The figure shows three views and two pictorial views of one solid part (mm, origin at its lowest corner). Answer the questions. A direction names the side the tool comes from. Coordinates: 2 decimals unless noted, no trailing zeros. Write each loop counter-clockwise with the first axis right and the second up, starting at its lowest first coordinate (ties: lowest second). Pieces come first, ordered by that corner, then holes. Notation, with made-up numbers: M 36.25,59 L 51.25,59 A20 ccw 51.25,75 Z; hole C -18.5,71.25 d2. An arc over 180 degrees is marked long. Answer as CSV lines item,"result".
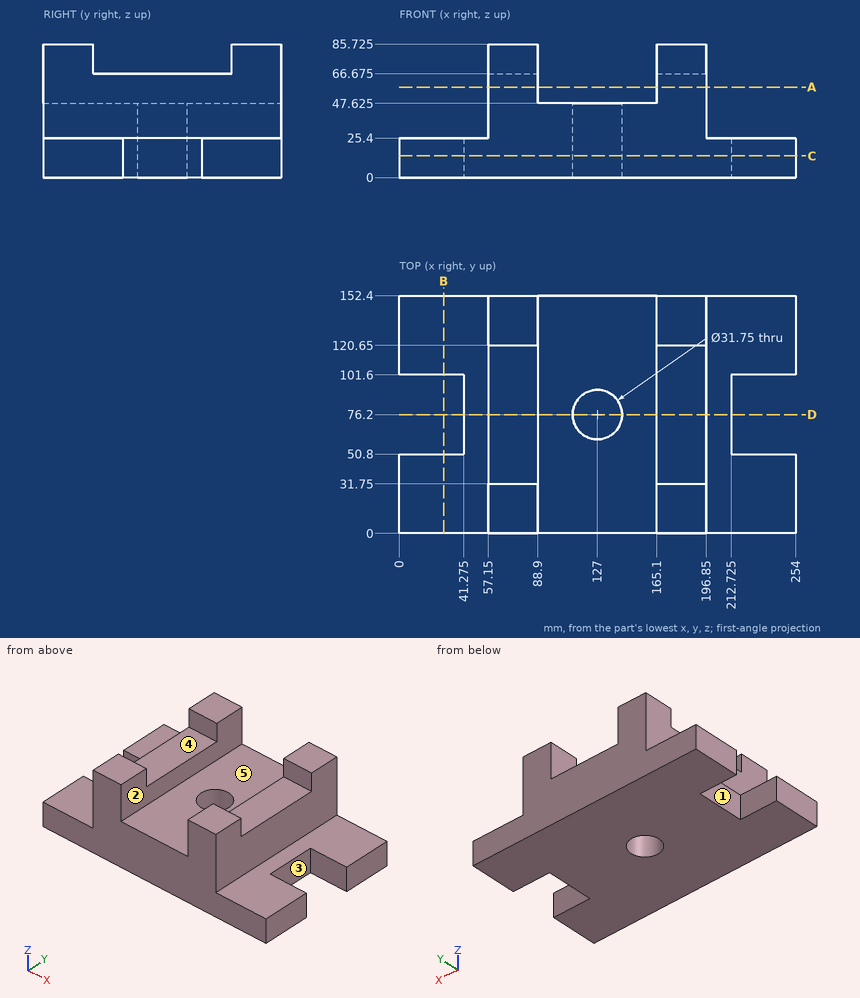
Q1. Straight lines are drawn through the part: line 1 (X direction, y = 76.2, z = 28) (3 decimals); line 2 (X direction, y = 88, z = 50.5); line 3 (Y direction, x = 127, z = 30) (3 decimals). For each, find the intervals that lie inside material, in ascending order.
Output:
line 1,"57.15 to 111.125, 142.875 to 196.85"
line 2,"57.15 to 88.9, 165.1 to 196.85"
line 3,"0 to 60.325, 92.075 to 152.4"
Q2. For the marked faces 1, 2 and 3, determine the directions among +Z, -Z, +X, -X, +Y, -Y from which every point of the face is accessible in a straight line to the end or side of a thin tool.
Output:
face 1,"+Z, -Z, -X"
face 2,"+Z, +Y, -Y"
face 3,"+Z, -Z, +X"
Q3. Flat-ended cylindrical pins translate along their axes: pin 1 Ø18 at (y, z) = (62, 40.5) entering from +X; pin 2 Ø1.5 at (y, z) = (94, 51.5) entering from -X; pin 3 Ø12.5 at (y, z) = (75.5, 15.5) entering from -X (3 decimals). Find the tip coordinate at first contact, or state that the pin passes through.
Output:
pin 1,"x = 196.85"
pin 2,"x = 57.15"
pin 3,"x = 41.275"
Q4. Find section C-C (z = 14). Give the vertices of the cut face in (x, y) (3 decimals), and give its area (3 significant figures).
Output:
outline,"M 0,0 L 254,0 L 254,50.8 L 212.725,50.8 L 212.725,101.6 L 254,101.6 L 254,152.4 L 0,152.4 L 0,101.6 L 41.275,101.6 L 41.275,50.8 L 0,50.8 Z; hole C 127,76.2 d31.75"
area,"33,700 mm2"
Q5. Find section A-A (z = 58). Give the vertices of the cut face in (x, y).
Output:
outline,"M 57.15,0 L 88.9,0 L 88.9,152.4 L 57.15,152.4 Z; M 165.1,0 L 196.85,0 L 196.85,152.4 L 165.1,152.4 Z"
Q6. The mould has two halves that part along Y. Classify the marked faces 4 and 5: pulls with the +Y half, pulls with the -Y half, needs draft (parallel to the pull), parting line crosses it, or undercut.
Output:
face 4,"undercut"
face 5,"needs draft"
Q7. Find section B-B (x = 28.5). Give the vertices of the cut face in (y, z), and give its area (3 significant figures).
Output:
outline,"M 0,0 L 50.8,0 L 50.8,25.4 L 0,25.4 Z; M 101.6,0 L 152.4,0 L 152.4,25.4 L 101.6,25.4 Z"
area,"2,580 mm2"
Q8. Find section D-D (y = 76.2). Give the vertices of the cut face in (x, z) (3 decimals).
Output:
outline,"M 41.275,0 L 111.125,0 L 111.125,47.625 L 88.9,47.625 L 88.9,66.675 L 57.15,66.675 L 57.15,25.4 L 41.275,25.4 Z; M 142.875,0 L 212.725,0 L 212.725,25.4 L 196.85,25.4 L 196.85,66.675 L 165.1,66.675 L 165.1,47.625 L 142.875,47.625 Z"
